from build123d import *

# Parameters (mm, degrees)
F0_R     = 32.890522
F0_R_2   = 11.576292
F1_DEPTH = 25.4


with BuildPart() as f1:
    # F0 (on Top) → F1 (new body)
    with BuildSketch(Plane.XY):
        with Locations((36.280491, 36.996896)):
            Circle(F0_R)
        with BuildLine():
            ThreePointArc((48.881385, 10.403025), (35.940113, 7.570706), (23.067818, 10.701616))
            Line((23.067818, 10.701616), (23.067818, 19.783714))
            ThreePointArc((23.067818, 19.783714), (35.696865, 12.074644), (48.881385, 18.78963))
            Line((48.881385, 18.78963), (48.881385, 10.403025))
        make_face(mode=Mode.SUBTRACT)
        with BuildLine():
            Line((19.511687, 42.886119), (19.511687, 12.813768))
            ThreePointArc((19.511687, 12.813768), (6.89469, 35.41855), (17.017825, 59.244731))
            Line((17.017825, 59.244731), (17.017825, 46.268191))
            Line((17.017825, 46.268191), (19.511687, 42.886119))
        make_face(mode=Mode.SUBTRACT)
        with Locations((36.280491, 27.229772)):
            Circle(F0_R_2, mode=Mode.SUBTRACT)
        with BuildLine():
            Line((53.049296, 42.886119), (55.543158, 46.268191))
            Line((55.543158, 46.268191), (55.543158, 59.244731))
            ThreePointArc((55.543158, 59.244731), (65.666293, 35.41855), (53.049296, 12.813768))
            Line((53.049296, 12.813768), (53.049296, 42.886119))
        make_face(mode=Mode.SUBTRACT)
        with BuildLine():
            Line((20.1381, 49.27608), (20.1381, 61.602581))
            ThreePointArc((20.1381, 61.602581), (36.280491, 66.425054), (52.422883, 61.602581))
            Line((52.422883, 61.602581), (52.422883, 49.27608))
            Line((52.422883, 49.27608), (48.945498, 44.046022))
            Line((48.945498, 44.046022), (48.945498, 35.573399))
            ThreePointArc((48.945498, 35.573399), (36.280491, 42.396133), (23.615485, 35.573399))
            Line((23.615485, 35.573399), (23.615485, 44.046022))
            Line((23.615485, 44.046022), (20.1381, 49.27608))
        make_face(mode=Mode.SUBTRACT)
    extrude(amount=F1_DEPTH)


solid = f1.part
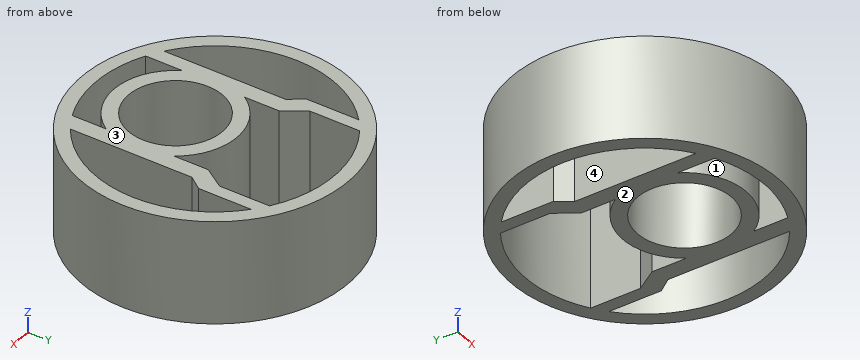
Work out the finished part from the listing and answer in its coordinate system (mm). Face numbers are marked on the shaded views. A direction names the side the tool comes from. Coordinates: 2 decimals unless noted, no trailing zeros. Write each loop counter-clockwise with the first axis right and the second up, starting at its lowest first coordinate (ties: lowest second). Pieces come first, ordered by that corner, then holes. Notation, with made-up numbers: M 28.25,5 L 46.25,5 A29 cw 46.25,44 Z; hole C 27.5,-6 d5. An arc over 180 degrees is marked long. Answer as CSV lines item,"result". Start each with the question number.
Item 1: Determine the mould class of the marked faces 1 and 2 for opening direction X: released by +X, released by -X, zero draft, split by the parting line, or undercut.
Item 2: A tool of negligible diameter and unlimited length cuts with its end or side. For the marked faces 3 and 4, from which of +Z, -Z, +X, -X, +Y, -Y can it reach the whole face along a straight path? Write none if from no direction.
Item 3: Consider L1, parallel to Y at x = 32, z = 2.5; L2, parallel to Y at x = 31, z = 22.75; L3, parallel to X at y = 33, z = 7. Determine where each line is inside the solid, lowest interval first.
Item 4: Section C-C on x = 12.5 is taken. Write down the section's boundary in (y, z), and give its area (3 significant figures).
Item 5: Section D-D on z = 19.5 is taken. Write down the section's boundary in (x, y), and give its area (3 significant figures).
Item 6: Section B-B on x = 42 is taken. Write down the section's boundary in (y, z), and give its area (3 significant figures).
Item 7: Section A-A on y = 55.5 is taken. Write down the section's boundary in (x, z), and give its area (3 significant figures).
Item 8: Flat-ended cylindrical pins translate along their axes: P1, Ø10, axis at y = 58, z = 8.5, coming from the -X side; P2, Ø6.5, axis at y = 15.5, z = 11.5, coming from the -X side; P3, Ø4, axis at y = 51, z = 15, coming from the +X side. Find the tip coordinate at first contact, or state that the pin passes through.
Checks:
1,face 1,"undercut"
1,face 2,"zero draft"
2,face 3,"+Z, +X, -X, +Y, -Y"
2,face 4,"+Z, -Z"
3,L1,"y = 4.39 to 7.88, 12.68 to 16.47, 37.99 to 41.78, 66.11 to 69.61"
3,L2,"y = 4.53 to 8.05, 13.01 to 16.93, 37.53 to 41.45, 65.95 to 69.46"
3,L3,"x = 3.63 to 7.13, 19.51 to 26.24, 46.32 to 53.05, 65.44 to 68.93"
4,outline,"M 14.28,0 L 19.66,0 L 19.66,25.4 L 14.28,25.4 Z; M 54.33,0 L 59.72,0 L 59.72,25.4 L 54.33,25.4 Z"
4,area,"274 mm²"
5,outline,"C 36.28,37 d65.78; hole M 17.02,46.27 L 17.02,59.24 A29.43 ccw 19.51,12.81 L 19.51,42.89 Z; hole M 20.14,49.28 L 23.62,44.05 L 23.62,35.57 A15.17 cw 48.95,35.57 L 48.95,44.05 L 52.42,49.28 L 52.42,61.6 A29.43 ccw 20.14,61.6 Z; hole M 23.07,10.7 A29.43 ccw 48.88,10.4 L 48.88,18.79 A15.17 cw 23.07,19.78 Z; hole C 36.28,27.23 d23.15; hole M 53.05,12.81 A29.43 ccw 55.54,59.24 L 55.54,46.27 L 53.05,42.89 Z"
5,area,"1,300 mm²"
6,outline,"M 4.61,0 L 8.13,0 L 8.13,25.4 L 4.61,25.4 Z; M 13.18,0 L 17.17,0 L 17.17,25.4 L 13.18,25.4 Z; M 37.29,0 L 41.28,0 L 41.28,25.4 L 37.29,25.4 Z; M 65.86,0 L 69.39,0 L 69.39,25.4 L 65.86,25.4 Z"
6,area,"381 mm²"
7,outline,"M 9.09,0 L 13.4,0 L 13.4,25.4 L 9.09,25.4 Z; M 17.02,0 L 20.14,0 L 20.14,25.4 L 17.02,25.4 Z; M 52.42,0 L 55.54,0 L 55.54,25.4 L 52.42,25.4 Z; M 59.16,0 L 63.47,0 L 63.47,25.4 L 59.16,25.4 Z"
7,area,"377 mm²"
8,P1,"stops at x = 7.55"
8,P2,"stops at x = 8.92"
8,P3,"stops at x = 66.9"
